Design review of the part built by this model. Coordinates are the model's own, in mm. Face numbers are marked on the shaded views. A direction names the side the tool comes from. Round coordinates to 2 decimals unless told otherwise and drop trailing zeros. Loops run counter-clockwise (first coordinate to the right, second up) from the corner with the lowest first, then second, coordinate; pieces in that order, holes last. Notation, with made-up numbers: (87.5, -34.5) - (141.5, -34.5) arc R16 cw to (141.5, -16.5) - close; hole circle Ø7 at (15.25, -35). An arc over 180 degrees is marked (long way). One line per question, with ' | ' between items. Start each with the question number.
from build123d import *

# Parameters (mm, degrees)
SKETCH_W        = 200
SKETCH_H        = 200
PAD_DEPTH       = 100
SKETCH001_W     = 195
SKETCH001_H     = 195
POCKET_DEPTH    = 98
SKETCH002_W     = 175
SKETCH002_H     = 70
POCKET001_DEPTH = 25


with BuildPart() as part:
    # Sketch → Pad (new body)
    with BuildSketch(Plane.XY):
        Rectangle(SKETCH_W, SKETCH_H)
    extrude(amount=PAD_DEPTH)

    # Sketch001 (on Face5 of Pad) → Pocket (cut)
    with BuildSketch(Plane(origin=(0, 0, 0), x_dir=(1, 0, 0), z_dir=(0, 0, -1))):
        Rectangle(SKETCH001_W, SKETCH001_H)
    extrude(amount=-POCKET_DEPTH, mode=Mode.SUBTRACT)

    # Sketch002 (on Face6 of Pocket) → Pocket001 (cut)
    with BuildSketch(Plane.XZ.offset(100)):
        with Locations((0, 35)):
            Rectangle(SKETCH002_W, SKETCH002_H)
    extrude(amount=-POCKET001_DEPTH, mode=Mode.SUBTRACT)


solid = part.part
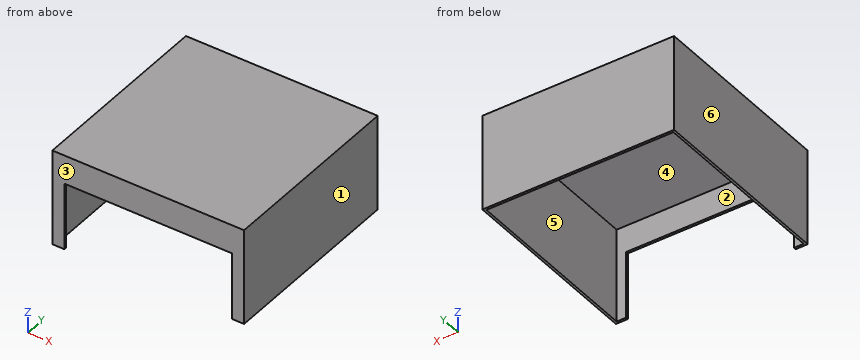
1. Take a section at A-A, the plane y = -24. Give the boundary of the cut face in (x, z), then the cut area to 3 significant figures.
2. Clearance check with flat-ended pins moving along their axes: P1, Ø2, axis at x = 62.5, y = -57.5, coming from the -Z side; P2, Ø3, axis at x = -23.5, y = -99, coming from the -Z side; P3, Ø10, axis at x = 12.5, z = 30.5, coming from the -Y side. State where each tip first meets the part, or that it passes through.
3. Take a section at B-B, the plane z = 39. Give the boundary of the cut face in (x, y), then the cut area to 3 significant figures.
4. Take a section at C-C, the plane x = 11. Give the boundary of the cut face in (y, z), then the cut area to 3 significant figures.
5. The part is to be moulded in two halves that separate along Y. For the marked faces 1, 2, 3 and 4, say which applies: pulls with the +Y half, pulls with the -Y half, needs draft (parallel to the pull), parting line crosses it, or undercut.
6. Machinability: for the marked faces 5 and 6, which of the approach directions +Z, -Z, +X, -X, +Y, -Y give a long, thin tool a straight path to every point of the face, cutting with its end or side? Answer none if there is none.
7. To check wall thickness, follow line 1 along X through (y, z) = (36.5, 78.5); line 2 along Y through (x, z) = (-82, 27); line 3 along Z through (x, y) = (-60.5, -87). State the ranges of each line that lie inside material, in increasing order.
Answer list:
1) outline: (-100, 0) - (-97.5, 0) - (-97.5, 98) - (97.5, 98) - (97.5, 0) - (100, 0) - (100, 100) - (-100, 100) - close | area: 890 mm²
2) P1: stops at z = 98 | P2: stops at z = 70 | P3: stops at y = 97.5
3) outline: (-100, -100) - (-87.5, -100) - (-87.5, -97.5) - (-97.5, -97.5) - (-97.5, 97.5) - (97.5, 97.5) - (97.5, -97.5) - (87.5, -97.5) - (87.5, -100) - (100, -100) - (100, 100) - (-100, 100) - close | area: 1,540 mm²
4) outline: (-100, 70) - (-97.5, 70) - (-97.5, 98) - (97.5, 98) - (97.5, 0) - (100, 0) - (100, 100) - (-100, 100) - close | area: 715 mm²
5) face 1: needs draft | face 2: undercut | face 3: pulls with the -Y half | face 4: undercut
6) face 5: -Z | face 6: +Z, -Z, -X, +Y, -Y
7) line 1: x = -100 to -97.5, 97.5 to 100 | line 2: y = 97.5 to 100 | line 3: z = 98 to 100
